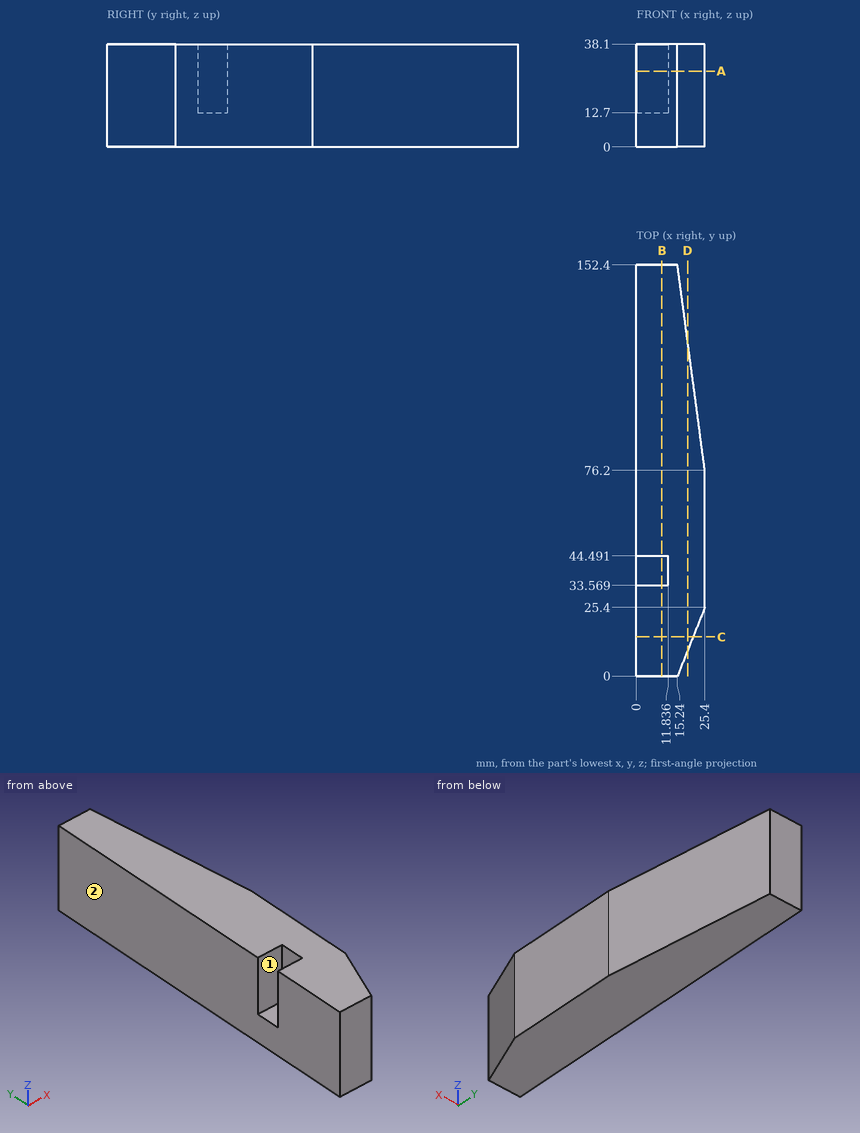
For this review, use the dimensioned drawing (mm, ordinates from the lowest corner) and the shaded views. A direction names the side the tool comes from. Coordinates: 2 decimals unless noted, no trailing zeros. Loops run counter-clockwise (first coordinate to the right, second up) from the corner with the lowest first, then second, coordinate; pieces in that order, holes last. Notation, with made-up numbers: (15, 35.5) -> (21, 35.5) arc R23 cw to (21, 49.5) -> close; hole circle Ø9 at (86.25, -8). An arc over 180 degrees is marked (long way). Return JSON: item names as keys, results as strings. Group by question number.
(1) Consider section A-A, the plane z = 28. Give the boundary of the cut face in (x, y) (1 decimal).
(2) Tool access review of the marked faces 1 and 2: name each direction out of +Z, -Z, +X, -X, +Y, -Y from which nothing blocks a thin tool from reaching the whole face with its end or side.
(3) Consider section C-C, the plane y = 14.5. Give the boundary of the cut face in (x, z).
(4) For pin 1 Ø3.5 at (x, y) = (4, 41.5) entering from +Z; pin 2 Ø3.5 at (y, z) = (40.5, 20) entering from -X, all flat-tipped, find the tip position at first contact; note any pin that passes through.
(5) Consider section D-D, the plane x = 19. Give the boundary of the cut face in (y, z).
(6) To check wall thickness, follow L1, parallel to Y at x = 8.5, z = 32; L2, parallel to X at y = 117, z = 2; L3, parallel to X at y = 117.5, z = 32. State the ranges of each line that lie inside material, in increasing order.
(7) Consider section B-B, the plane x = 9.5. Give the boundary of the cut face in (y, z).
Results below:
{
 "1": {"outline": "(0, 0) -> (15.2, 0) -> (25.4, 25.4) -> (25.4, 76.2) -> (15.2, 152.4) -> (0, 152.4) -> (0, 44.5) -> (11.8, 44.5) -> (11.8, 33.6) -> (0, 33.6) -> close"},
 "2": {"face 1": "+Z, -X", "face 2": "+Z, -Z, -X, +Y, -Y"},
 "3": {"outline": "(0, 0) -> (21.04, 0) -> (21.04, 38.1) -> (0, 38.1) -> close"},
 "4": {"pin 1": "stops at z = 12.7", "pin 2": "stops at x = 11.84"},
 "5": {"outline": "(9.4, 0) -> (124.2, 0) -> (124.2, 38.1) -> (9.4, 38.1) -> close"},
 "6": {"L1": "y = 0 to 33.57, 44.49 to 152.4", "L2": "x = 0 to 19.96", "L3": "x = 0 to 19.89"},
 "7": {"outline": "(0, 0) -> (152.4, 0) -> (152.4, 38.1) -> (44.49, 38.1) -> (44.49, 12.7) -> (33.57, 12.7) -> (33.57, 38.1) -> (0, 38.1) -> close"}
}
